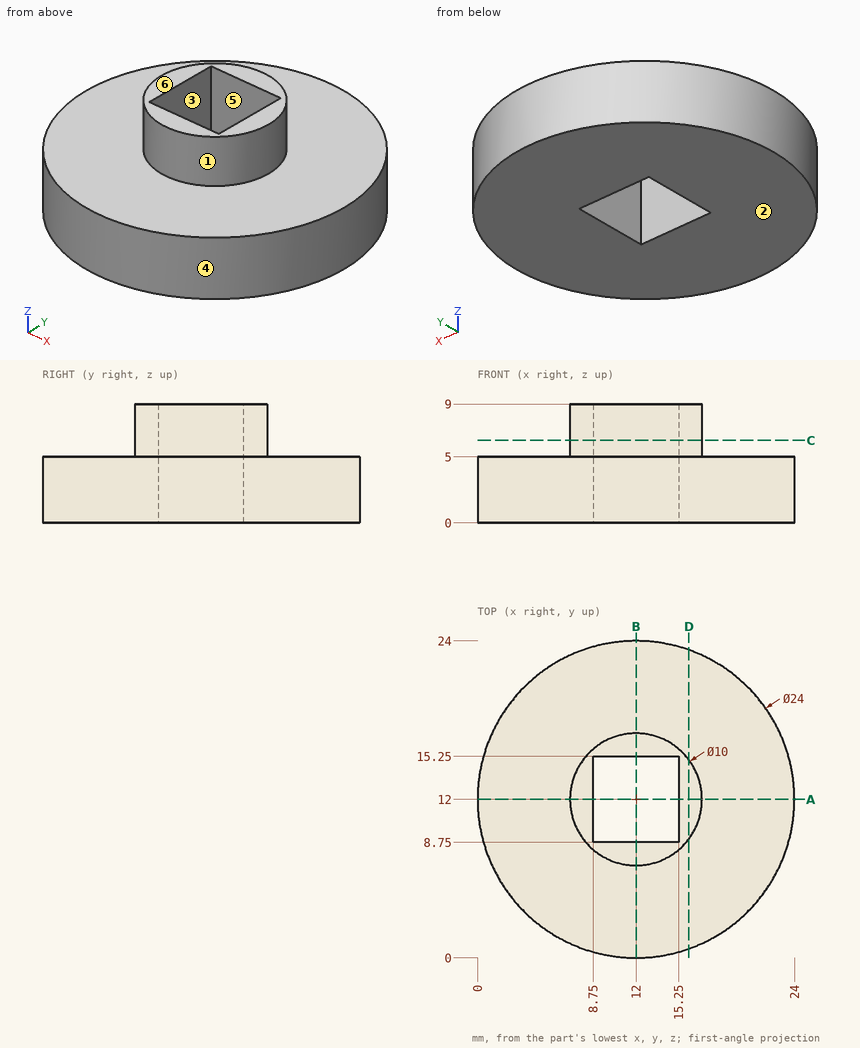
For this review, use the dimensioned drawing (mm, ordinates from the lowest corner) and the shaded views. A direction names the side the tool comes from. Give positions to 0.01 mm unless a question says otherwise; leave off trailing zeros. Write each loop counter-clockwise with the first axis right and the second up, starting at its lowest first coordinate (ties: lowest second). Pieces come first, ordered by that corner, then holes. Notation, with made-up numbers: M -26,-22 L 6,-22 A29 cw 6,4 Z; hole C -16,-19.75 d7. An arc over 180 degrees is marked long. Write item = value, one per line. Start each with the question number.
Q1. Clearance check with flat-ended pins moving along their axes: pin 1 (4 mm diameter, centred on y = 14.5, z = 7.5, fed in from +X); pin 2 (1 mm diameter, centred on x = 11.5, y = 2.5, fed in from +Z). State where each tip first meets the part, or that it passes through.
Q2. For line 1 (Z direction, x = 19.75, y = 11); line 2 (X direction, y = 14, z = 7); line 3 (X direction, y = 14.75, z = 2.75), list the stretches that pass through material, from the lowest coordinate up.
Q3. Machinability: for the marked faces 1, 2 and 3, which of the approach directions +Z, -Z, +X, -X, +Y, -Y give a long, thin tool a straight path to every point of the face, cutting with its end or side? Answer none if there is none.
Q4. We need section A-A (y = 12). State the section outline as (x, z) points.
Q5. We need section D-D (x = 16). State the section outline as (y, z) points.
Q6. We need section C-C (z = 6.25). State the section outline as (x, y) points, plus the area to 3 significant figures.
Q7. Mouldability with a two-part tool opening along Y and no side actions: class the marked faces 4, 5 and 6 as released by +Y, released by -Y, zero draft, split by the parting line, or undercut.
Result set:
q1.pin_1 = 16.97
q1.pin_2 = 5
q2.line_1 = 0 to 5
q2.line_2 = 7.42 to 8.75, 15.25 to 16.58
q2.line_3 = 0.32 to 8.75, 15.25 to 23.68
q3.face_1 = +Z
q3.face_2 = -Z, +X, -X, +Y, -Y
q3.face_3 = +Z, -Z
q4.outline = M 0,0 L 8.75,0 L 8.75,9 L 7,9 L 7,5 L 0,5 Z; M 15.25,0 L 24,0 L 24,5 L 17,5 L 17,9 L 15.25,9 Z
q5.outline = M 0.69,0 L 23.31,0 L 23.31,5 L 15,5 L 15,9 L 9,9 L 9,5 L 0.69,5 Z
q6.outline = C 12,12 d10; hole M 8.75,8.75 L 15.25,8.75 L 15.25,15.25 L 8.75,15.25 Z
q6.area = 36.3 mm2
q7.face_4 = split by the parting line
q7.face_5 = undercut
q7.face_6 = zero draft
